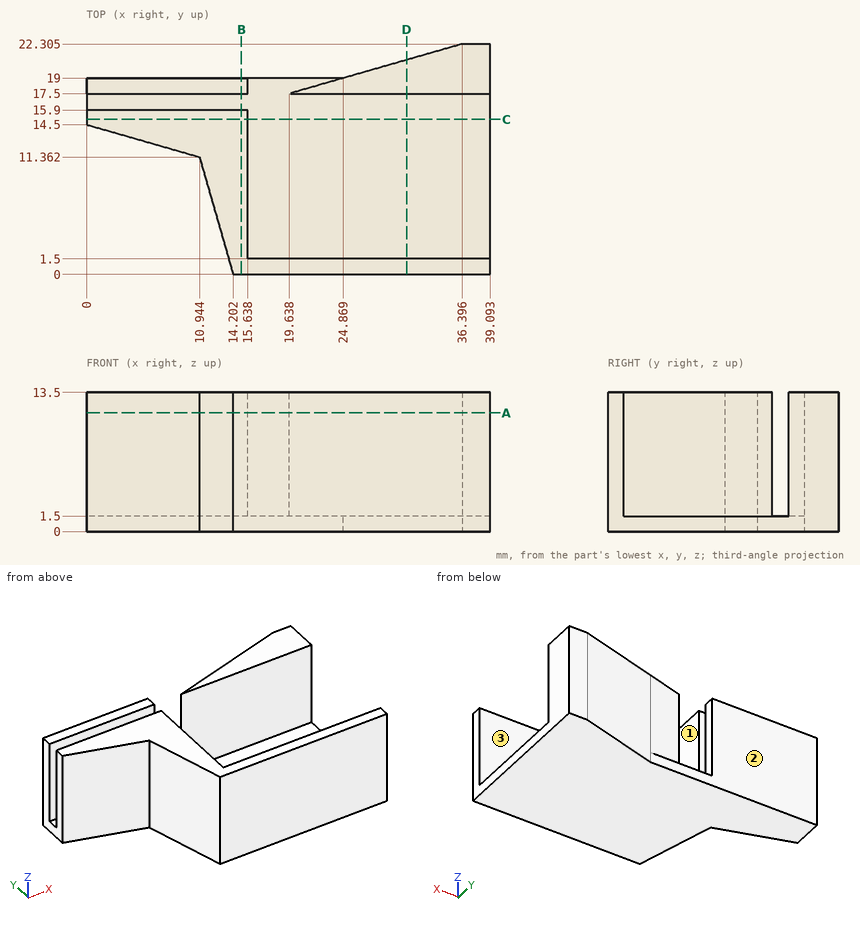
Design review of the part shown in the three views and the two pictorial views. Dimensions are in mm from the part's minimum x, y and z. A direction names the side the tool comes from. Give positions to 0.01 mm unless a question says otherwise; leave off trailing zeros. Loops run counter-clockwise (first coordinate to the right, second up) from the corner with the lowest first, then second, coordinate; pieces in that order, holes last. Notation, with made-up numbers: M -26.5,-35.75 L -6.5,-35.75 A33 cw -6.5,-5.75 Z; hole C 50,65 d3. An arc over 180 degrees is marked long. Answer as a JSON object with one key per item and string values.
Item 1: We need section B-B (x = 15). State the section outline as (y, z) points, and give its area (3 significant figures).
Output values:
{"outline": "M 0,0 L 19,0 L 19,13.5 L 17.5,13.5 L 17.5,1.5 L 15.9,1.5 L 15.9,13.5 L 0,13.5 Z", "area": "237 mm2"}
Item 2: We need section C-C (y = 15). State the section outline as (x, z) points.
Output values:
{"outline": "M 0,0 L 39.09,0 L 39.09,1.5 L 15.64,1.5 L 15.64,13.5 L 0,13.5 Z"}
Item 3: For P1, Ø6, axis at x = 31, z = 5.5, coming from the +Y side; P2, Ø3.5, axis at y = 9.5, z = 10, coming from the +X side; P3, Ø6, axis at x = 8, z = 5.5, coming from the +Y side, all flat-tipped, find the tip position at first contact; note any pin that passes through.
Output values:
{"P1": "stops at y = 21.62", "P2": "stops at x = 15.64", "P3": "stops at y = 19"}
Item 4: Machinability: for the marked faces 1, 2 and 3, which of the approach directions +Z, -Z, +X, -X, +Y, -Y give a long, thin tool a straight path to every point of the face, cutting with its end or side? Answer none if there is none.
Output values:
{"face 1": "+Z, +X, +Y", "face 2": "+Z, -Z, -X, +Y", "face 3": "+Z, +X"}
Item 5: We need section D-D (x = 31). State the section outline as (y, z) points.
Output values:
{"outline": "M 0,0 L 20.76,0 L 20.76,13.5 L 17.5,13.5 L 17.5,1.5 L 1.5,1.5 L 1.5,13.5 L 0,13.5 Z"}
Item 6: We need section A-A (z = 11.5). State the section outline as (x, y) points (1 decimal).
Output values:
{"outline": "M 0,14.5 L 10.9,11.4 L 14.2,0 L 39.1,0 L 39.1,1.5 L 15.6,1.5 L 15.6,15.9 L 0,15.9 Z; M 0,17.5 L 15.6,17.5 L 15.6,19 L 0,19 Z; M 19.6,17.5 L 39.1,17.5 L 39.1,22.3 L 36.4,22.3 Z"}
Item 7: Wall thickness on line 1 along Y through (x, z) = (37.5, 3.5) (1 decimal); line 2 along Y through (x, z) = (7, 6); line 3 along Z through (x, y) = (23, 15): over which ranges is each line inside the solid? List them lowest first.
Output values:
{"line 1": "y = 0 to 1.5, 17.5 to 22.3", "line 2": "y = 12.49 to 15.9, 17.5 to 19", "line 3": "z = 0 to 1.5"}
